Verification items for the finished model (mm, model axes). Face numbers are marked on the shaded views. A direction names the side the tool comes from. Coordinates: 2 decimals unless noted, no trailing zeros. Order: outer loops, then holes, each group sorted by start corner. A loop starts at its lowest first (then second) coordinate and runs counter-clockwise, first axis right, second up.
Q1. Depth check by flat-ended pin: P1, Ø4, axis at x = 5, z = -85.5, coming from the +Y side; P2, Ø22, axis at x = -24, z = -67, coming from the +Y side; P3, Ø12, axis at y = 14, z = -9.5, coming from the -X side. Enter the tip coordinate at first touch or a pass-through.
Q2. Cross-section at A-A, the plane y = 14. Record the boundary of the cut face in (x, z), and give its area (3 significant figures).
Q3. Set-up check for the marked faces 1, 2 and 3: record each of +Z, -Z, +X, -X, +Y, -Y from which the full face is reachable in a straight line by a thin tool's end or side.
Q4. Thickness scan on line 1 (X direction, y = 2.15, z = -67.5); line 2 (X direction, y = 1, z = -86); line 3 (X direction, y = 11.5, z = -56). Record the ranges inside material, lowest first.
Q5. Cross-section at B-B, the plane z = -38. Record the boundary of the cut face in (x, y).
from build123d import *

# Parameters (mm, degrees)
BOSS_EXTRUDE1_DEPTH = 30
BOSS_EXTRUDE2_DEPTH = 2
SKETCH5_R           = 12
SKETCH5_R_2         = 10
BOSS_EXTRUDE3_DEPTH = 7
SKETCH6_W           = 8
SKETCH6_H           = 8
BOSS_EXTRUDE4_DEPTH = 10
CUT_EXTRUDE1_START  = 10
CUT_EXTRUDE1_DEPTH  = 2.2
FILLET1_R           = 2
SKETCH8_W           = 10
SKETCH8_H           = 10
CUT_EXTRUDE3_DEPTH  = 122.128031438


with BuildPart() as part:
    # Sketch2 → Boss-Extrude1 (new body)
    with BuildSketch(Plane(origin=(0, 0, 0), x_dir=(1, 0, 0), z_dir=(0, 1, 0))):
        with BuildLine():
            Line((72, 2), (72, 88))
            ThreePointArc((72, 88), (70.828427125, 90.828427125), (68, 92))
            Line((68, 92), (-48, 92))
            ThreePointArc((-48, 92), (-50.828427125, 90.828427125), (-52, 88))
            Line((-52, 88), (-52, 47))
            ThreePointArc((-52, 47), (-50.828427125, 44.171572875), (-48, 43))
            Line((-48, 43), (-2, 43))
            Line((-2, 43), (-2, 2))
            ThreePointArc((-2, 2), (-0.828427125, -0.828427125), (2, -2))
            Line((2, -2), (68, -2))
            ThreePointArc((68, -2), (70.828427125, -0.828427125), (72, 2))
        make_face()
        with BuildLine():
            Line((70, 2), (70, 88))
            ThreePointArc((70, 88), (69.414213562, 89.414213562), (68, 90))
            Line((68, 90), (-48, 90))
            ThreePointArc((-48, 90), (-49.414213562, 89.414213562), (-50, 88))
            Line((-50, 88), (-50, 47))
            ThreePointArc((-50, 47), (-49.414213562, 45.585786438), (-48, 45))
            Line((-48, 45), (-2, 45))
            ThreePointArc((-2, 45), (-0.585786438, 44.414213562), (0, 43))
            Line((0, 43), (0, 2))
            ThreePointArc((0, 2), (0.585786438, 0.585786438), (2, 0))
            Line((2, 0), (68, 0))
            ThreePointArc((68, 0), (69.414213562, 0.585786438), (70, 2))
        make_face(mode=Mode.SUBTRACT)
    extrude(amount=BOSS_EXTRUDE1_DEPTH)



with BuildPart() as body_2:
    # Sketch3 → Boss-Extrude2 (new body)
    # profile 1 of 2: a face of its own
    with BuildSketch(Plane(origin=(0, 0, 0), x_dir=(1, 0, 0), z_dir=(0, 1, 0))):
        with BuildLine():
            Line((-48, 92), (68, 92))
            ThreePointArc((68, 92), (70.828427125, 90.828427125), (72, 88))
            Line((72, 88), (72, 2))
            ThreePointArc((72, 2), (70.828427125, -0.828427125), (68, -2))
            Line((68, -2), (2, -2))
            ThreePointArc((2, -2), (-0.828427125, -0.828427125), (-2, 2))
            Line((-2, 2), (-2, 43))
            Line((-2, 43), (-48, 43))
            ThreePointArc((-48, 43), (-50.828427125, 44.171572875), (-52, 47))
            Line((-52, 47), (-52, 88))
            ThreePointArc((-52, 88), (-50.828427125, 90.828427125), (-48, 92))
        make_face()
        with BuildLine():
            Line((0, 43), (0, 2))
            ThreePointArc((0, 2), (0.585786438, 0.585786438), (2, 0))
            Line((2, 0), (68, 0))
            ThreePointArc((68, 0), (69.414213562, 0.585786438), (70, 2))
            Line((70, 2), (70, 88))
            ThreePointArc((70, 88), (69.414213562, 89.414213562), (68, 90))
            Line((68, 90), (-48, 90))
            ThreePointArc((-48, 90), (-49.414213562, 89.414213562), (-50, 88))
            Line((-50, 88), (-50, 47))
            ThreePointArc((-50, 47), (-49.414213562, 45.585786438), (-48, 45))
            Line((-48, 45), (-2, 45))
            ThreePointArc((-2, 45), (-0.585786438, 44.414213562), (0, 43))
        make_face(mode=Mode.SUBTRACT)
    # profile 2 of 2: a face of its own
    with BuildSketch(Plane(origin=(0, 0, 0), x_dir=(1, 0, 0), z_dir=(0, 1, 0))):
        with BuildLine():
            ThreePointArc((0, 43), (-0.585786438, 44.414213562), (-2, 45))
            Line((-2, 45), (-48, 45))
            ThreePointArc((-48, 45), (-49.414213562, 45.585786438), (-50, 47))
            Line((-50, 47), (-50, 88))
            ThreePointArc((-50, 88), (-49.414213562, 89.414213562), (-48, 90))
            Line((-48, 90), (68, 90))
            ThreePointArc((68, 90), (69.414213562, 89.414213562), (70, 88))
            Line((70, 88), (70, 2))
            ThreePointArc((70, 2), (69.414213562, 0.585786438), (68, 0))
            Line((68, 0), (2, 0))
            ThreePointArc((2, 0), (0.585786438, 0.585786438), (0, 2))
            Line((0, 2), (0, 43))
        make_face()
    extrude(amount=-BOSS_EXTRUDE2_DEPTH)


with BuildPart() as part_1:
    add(part.part)

    add(body_2.part)  # Boss-Extrude3 merges body 2
    # Sketch5 → Boss-Extrude3 (add)
    with BuildSketch(Plane(origin=(0, 0, 0), x_dir=(1, 0, 0), z_dir=(0, 1, 0))):
        with Locations(Location((-25, 67.5, 0), (0, 0, 270))):
            Circle(SKETCH5_R)
        with Locations(Location((-25, 67.5, 0), (0, 0, 270))):
            Circle(SKETCH5_R_2, mode=Mode.SUBTRACT)
    extrude(amount=BOSS_EXTRUDE3_DEPTH)

    # Sketch6 → Boss-Extrude4 (add)
    with BuildSketch(Plane(origin=(0, 0, 0), x_dir=(1, 0, 0), z_dir=(0, 1, 0))):
        with Locations((65, 85)):
            Rectangle(SKETCH6_W, SKETCH6_H)
        Polygon((60.857142857, 8), (68.857142857, 8), (68.857142857, 2), (67.357142857, 0.5), (60.857142857, 0.5), align=None)
        Polygon((9.142857143, 0.5), (9.142857143, 8), (1.142857143, 8), (1.142857143, 2), (2.642857143, 0.5), align=None)
        with Locations((5, 85)):
            Rectangle(SKETCH6_W, SKETCH6_H)
    extrude(amount=BOSS_EXTRUDE4_DEPTH)

    # Sketch7 → Cut-Extrude1 (cut)
    with BuildSketch(Plane(origin=(0, 0, 0), x_dir=(1, 0, 0), z_dir=(0, 1, 0)).offset(CUT_EXTRUDE1_START)):
        Polygon((2.4, 86.5011107), (2.4, 83.4988893), (5, 81.9977786), (7.6, 83.4988893), (7.6, 86.5011107), (5, 88.0022214), align=None)
        Polygon((2.4, 5.643967843), (2.4, 2.641746443), (5, 1.140635743), (7.6, 2.641746443), (7.6, 5.643967843), (5, 7.145078543), align=None)
        Polygon((65, 1.140635743), (62.4, 2.641746443), (62.4, 5.643967843), (65, 7.145078543), (67.6, 5.643967843), (67.6, 2.641746443), align=None)
        Polygon((62.4, 86.5011107), (65, 88.0022214), (67.6, 86.5011107), (67.6, 83.4988893), (65, 81.9977786), (62.4, 83.4988893), align=None)
    extrude(amount=-CUT_EXTRUDE1_DEPTH, mode=Mode.SUBTRACT)

    # Fillet1
    fillet1_edges = [part_1.edges().sort_by_distance(p)[0] for p in [
        (61, 5, -89),
        (61, 5, -81),
        (69, 5, -81),
        (69, 5, -89),
        (60.857142857, 5, -8),
        (60.857142857, 5, -0.5),
        (68.857142857, 5, -8),
        (9.142857143, 5, -8),
        (1.142857143, 5, -8),
        (9.142857143, 5, -0.5),
        (9, 5, -81),
        (9, 5, -89),
        (1, 5, -89),
        (1, 5, -81),
        (-2, 14, -43),
        (-25, 7, -77.5),
    ]]
    fillet(fillet1_edges, radius=FILLET1_R - 0.0001)  # a hair under: the kernel refuses the full size

    # Sketch8 → Cut-Extrude3 (cut, through all)
    with BuildSketch(Plane.XZ.offset(2)):
        with Locations((35, -7)):
            Rectangle(SKETCH8_W, SKETCH8_H)
    extrude(amount=-CUT_EXTRUDE3_DEPTH, mode=Mode.SUBTRACT)


solid = part_1.part
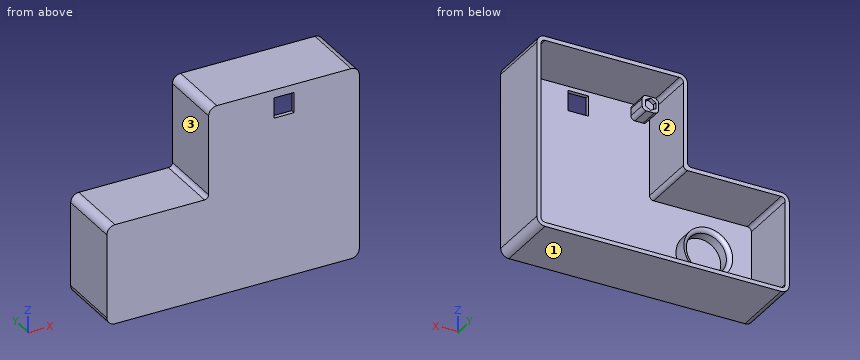
Check values:
1. P1: stops at y = 7.8
1. P2: stops at y = 7
1. P3: stops at x = -2
2. outline: (-52, -88) arc R4 ccw to (-48, -92) - (68, -92) arc R4 ccw to (72, -88) - (72, -2) arc R4 ccw to (68, 2) - (2, 2) arc R4 ccw to (-2, -2) - (-2, -41) arc R2 cw to (-4, -43) - (-48, -43) arc R4 ccw to (-52, -47) - close; hole (-50, -88) arc R2 ccw to (-48, -90) - (68, -90) arc R2 ccw to (70, -88) - (70, -2) arc R2 ccw to (68, 0) - (2, 0) arc R2 ccw to (0, -2) - (0, -43) arc R2 cw to (-2, -45) - (-48, -45) arc R2 ccw to (-50, -47) - close
2. area: 843 mm2
3. face 1: -Z, +X, -X, +Y, -Y
3. face 2: +Y
3. face 3: +Z, -X, +Y, -Y
4. line 1: x = -52 to -50, -37 to -35, -15 to -13, 70 to 72
4. line 2: x = -52 to -50, 1 to 9, 61 to 69, 70 to 72
4. line 3: x = -52 to -50, 70 to 72
5. outline: (-2, -2) - (72, -2) - (72, 30) - (70, 30) - (70, 0) - (0, 0) - (0, 30) - (-2, 30) - close
